```python
from build123d import *

# Parameters (mm, degrees)
EXTRUSION1_DEPTH        = 11
CONG_2_R                = 2
ESQUISSE2_R             = 4
ENL_V_MAT_EXTRU_1_DEPTH = 72.867934435


with BuildPart() as part:
    # Esquisse1 → Extrusion1 (new, symmetric)
    with BuildSketch(Plane.XY):
        with BuildLine():
            Line((0, 0), (37.484227511, 0))
            ThreePointArc((37.484227511, 0), (40.385390018, -0.430085888), (43.037002714, -1.683348779))
            Line((43.037002714, -1.683348779), (48.478769775, -5.316651221))
            ThreePointArc((48.478769775, -5.316651221), (51.130382471, -6.569914112), (54.031544979, -7))
            Line((54.031544979, -7), (70, -7))
            Line((70, -7), (70, -12))
            Line((70, -12), (52.515772489, -12))
            ThreePointArc((52.515772489, -12), (49.614609982, -11.569914112), (46.962997286, -10.316651221))
            Line((46.962997286, -10.316651221), (41.521230225, -6.683348779))
            ThreePointArc((41.521230225, -6.683348779), (38.869617529, -5.430085888), (35.968455021, -5))
            Line((35.968455021, -5), (0, -5))
            Line((0, -5), (0, 0))
        make_face()
    extrude(amount=EXTRUSION1_DEPTH, both=True)

    # Congé2
    cong_2_edges = [part.edges().sort_by_distance(p)[0] for p in [
        (38.869617529, -5.430085888, 11),
        (40.385390018, -0.430085888, -11),
        (45.757886245, -3.5, -11),
        (51.130382471, -6.569914112, -11),
        (62.015772489, -7, -11),
        (61.257886245, -12, -11),
        (49.614609982, -11.569914112, -11),
        (44.242113755, -8.5, -11),
        (44.242113755, -8.5, 11),
        (38.869617529, -5.430085888, -11),
        (17.984227511, -5, -11),
        (49.614609982, -11.569914112, 11),
        (61.257886245, -12, 11),
        (62.015772489, -7, 11),
        (51.130382471, -6.569914112, 11),
        (45.757886245, -3.5, 11),
        (40.385390018, -0.430085888, 11),
        (18.742113755, 0, 11),
        (17.984227511, -5, 11),
        (18.742113755, 0, -11),
    ]]
    fillet(cong_2_edges, radius=CONG_2_R)

    # Esquisse2 → Enlèv. mat.-Extru.1 (cut, through all)
    with BuildSketch(Plane(origin=(0, 0, 0), x_dir=(-1, 0, 0), z_dir=(0, 1, 0))):
        with Locations(Location((-10, 0, 0), (0, 0, 90))):
            Circle(ESQUISSE2_R)
    extrude(amount=-ENL_V_MAT_EXTRU_1_DEPTH, mode=Mode.SUBTRACT)

    # Esquisse3 → Enlèvement de matière-Révolution1 (revolve, cut)
    with BuildSketch(Plane.XY, mode=Mode.PRIVATE) as enl_vement_de_mati_re_r_volution1_sk:
        Polygon((65, -7), (65.881634904, -12), (60, -12), (60, -7), align=None)
    revolve(enl_vement_de_mati_re_r_volution1_sk.sketch.rotate(Axis((60, 1.983898021, 0), (0, -1, 0)), 90), axis=Axis((60, 1.983898021, 0), (0, -1, 0)), mode=Mode.SUBTRACT)


solid = part.part
```
Part model, mm, in its own coordinate system. A direction names the side the tool comes from. Round coordinates to 2 decimals unless told otherwise and drop trailing zeros. Loops run counter-clockwise (first coordinate to the right, second up) from the corner with the lowest first, then second, coordinate; pieces in that order, holes last.
Item 1: Mould opens along Z. For faces 1 (the face through (13.966, -2.465, -0.521)), 2 (the face through (61.14, -11.43, -10.4)), 3 (the face through (0, -3, 0)) say: +Z half, -Z half, draft (parallel to the pull), parting line (faces both ways), or undercut.
Item 2: Drop flat-ended pins along their axis: P1, Ø10, axis at x = 22, z = -0.5, coming from the -Y side; P2, Ø6, axis at x = 31.5, y = -9.5, coming from the -Z side; P3, Ø8, axis at x = 60, z = -1.5, coming from the +Y side; P4, Ø6, axis at y = -1.5, z = -3, coming from the +X side. Give the stop position or say it passes through.
Item 3: Cut at A-A, the plane z = 0. Give the cut face in (x, y).
Item 4: 3-axis set-ups, long thin cutter, end or side, ignore diameter. For faces 4 (the face through (19, -0.57, -10.4)), 5 (the face through (62.13, -7.6, 10.43)): which of +Z, -Z, +X, -X, +Y, -Y reach the whole face in a straight line?
Item 5: Drill centre lines: line 1 (Y direction, x = 12.5, z = -5.25); line 2 (X direction, y = -0.75, z = 1.5); line 3 (X direction, y = -4.5, z = 3.5). Where is each one in solid material? Low to high.
Item 6: Cut at D-D, the plane z = 7. Give the cut face in (x, y).
Item 7: Cut at C-C, the plane x = 10. Give the cut face in (y, z), then the cut area to 3 significant figures.
Item 8: Cut at B-B, the plane x = 60. Give the cut face in (y, z), then the cut area to 3 significant figures.
A:
1. face 1: undercut
1. face 2: -Z half
1. face 3: draft
2. P1: stops at y = -5
2. P2: passes through
2. P3: stops at y = -7
2. P4: stops at x = 47.26
3. outline: (0, -5) - (6, -5) - (6, 0) - (0, 0) - close; (14, -5) - (35.97, -5) arc R10 cw to (41.52, -6.68) - (46.96, -10.32) arc R10 ccw to (52.52, -12) - (54.12, -12) - (55, -7) - (54.03, -7) arc R10 cw to (48.48, -5.32) - (43.04, -1.68) arc R10 ccw to (37.48, 0) - (14, 0) - close; (65, -7) - (65.88, -12) - (70, -12) - (70, -7) - close
4. face 4: -Z, +X, -X, +Y
4. face 5: +Z, +X, +Y
5. line 1: y = -5 to 0
5. line 2: x = 0 to 6.29, 13.71 to 41.28
5. line 3: x = 0 to 8.06, 11.94 to 47.26
6. outline: (0, -5) - (35.97, -5) arc R10 cw to (41.52, -6.68) - (46.96, -10.32) arc R10 ccw to (52.52, -12) - (70, -12) - (70, -7) - (54.03, -7) arc R10 cw to (48.48, -5.32) - (43.04, -1.68) arc R10 ccw to (37.48, 0) - (0, 0) - close
7. outline: (-5, -9) arc R2 ccw to (-3, -11) - (-2, -11) arc R2 ccw to (0, -9) - (0, -4) - (-5, -4) - close; (-5, 4) - (0, 4) - (0, 9) arc R2 ccw to (-2, 11) - (-3, 11) arc R2 ccw to (-5, 9) - close
7. area: 66.6 mm2
8. outline: (-12, -9) arc R2 ccw to (-10, -11) - (-9, -11) arc R2 ccw to (-7, -9) - (-7, -5) - (-12, -5.88) - close; (-12, 5.88) - (-7, 5) - (-7, 9) arc R2 ccw to (-9, 11) - (-10, 11) arc R2 ccw to (-12, 9) - close
8. area: 52.2 mm2
